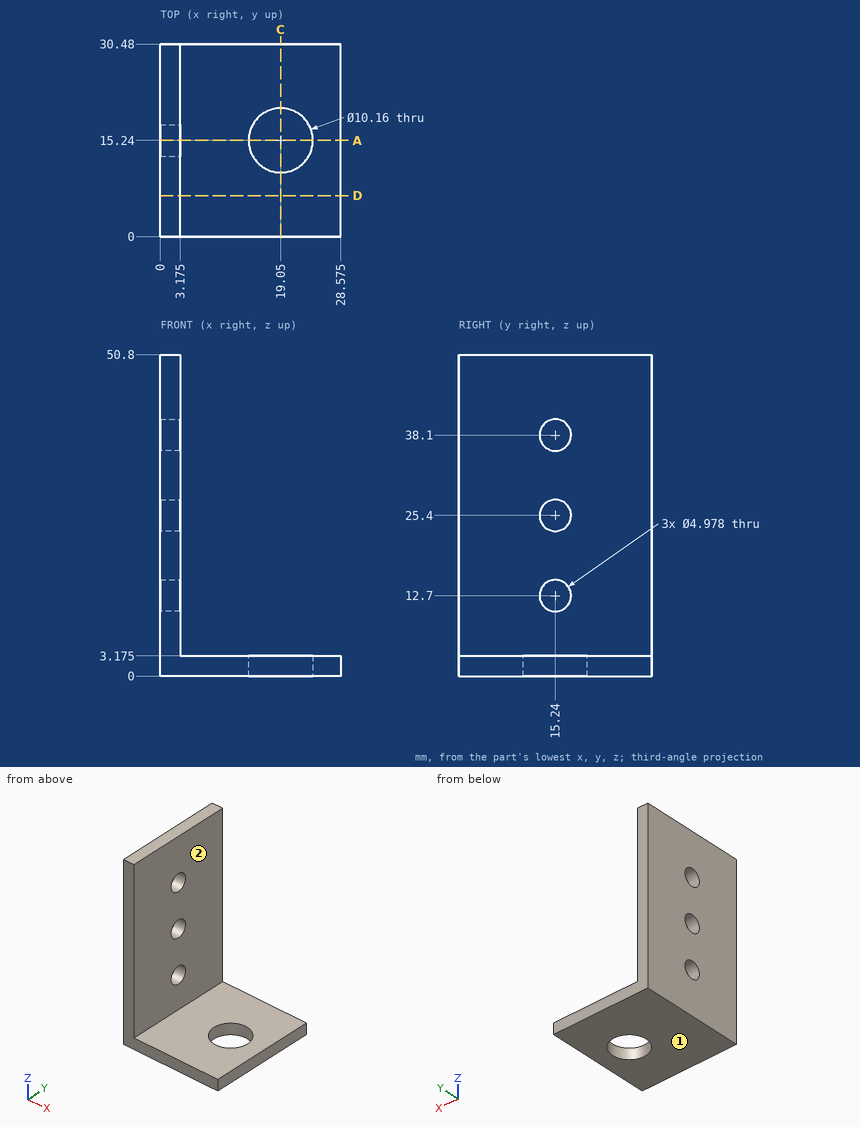
Job drawing, mm, ordinate dimensions from the low corner. One solid piece. A direction names the side the tool comes from. Round coordinates to 2 decimals unless told otherwise and drop trailing zeros. Loops run counter-clockwise (first coordinate to the right, second up) from the corner with the lowest first, then second, coordinate; pieces in that order, holes last. Notation, with made-up numbers: (-39.5, -14) -> (-19.5, -14) arc R16 cw to (-19.5, 13) -> close; hole circle Ø4 at (-36.5, 74.25). An arc over 180 degrees is marked (long way). One line per item, written item: value. Start each with the question number.
Q1. Drop flat-ended pins along their axis: pin 1 Ø4.5 at (y, z) = (15.24, 25.4) entering from -X; pin 2 Ø10 at (y, z) = (16, 34) entering from -X; pin 3 Ø7.5 at (x, y) = (20, 21) entering from +Z (3 decimals). Give the stop position or say it passes through.
Q2. Cut at D-D on y = 6.5. List the corners of the cut face in (x, z) (1 decimal), plus the area to 3 significant figures.
Q3. 3-axis set-ups, long thin cutter, end or side, ignore diameter. For the marked faces 1 and 2: which of +Z, -Z, +X, -X, +Y, -Y reach the whole face in a straight line?
Q4. Probe line 1 along Y through (x, z) = (0.8, 12.7); line 2 along X through (y, z) = (9, 46) (1 decimal); line 3 along Y through (x, z) = (19.05, 2.15). List the from-to ranges inside material, lowest first.
Q5. Cut at A-A on y = 15.24. List the corners of the cut face in (x, z) (1 decimal).
Q6. Cut at C-C on x = 19.05. List the corners of the cut face in (y, z) (1 decimal).
Computed:
1. pin 1: through
1. pin 2: x = 0
1. pin 3: z = 3.175
2. outline: (0, 0) -> (28.6, 0) -> (28.6, 3.2) -> (3.2, 3.2) -> (3.2, 50.8) -> (0, 50.8) -> close
2. area: 242 mm²
3. face 1: -Z, +X, -X, +Y, -Y
3. face 2: +Z, +X, +Y, -Y
4. line 1: 0 to 12.75, 17.73 to 30.48
4. line 2: 0 to 3.2
4. line 3: 0 to 10.16, 20.32 to 30.48
5. outline: (0, 0) -> (14, 0) -> (14, 3.2) -> (3.2, 3.2) -> (3.2, 10.2) -> (0, 10.2) -> close; (0, 15.2) -> (3.2, 15.2) -> (3.2, 22.9) -> (0, 22.9) -> close; (0, 27.9) -> (3.2, 27.9) -> (3.2, 35.6) -> (0, 35.6) -> close; (0, 40.6) -> (3.2, 40.6) -> (3.2, 50.8) -> (0, 50.8) -> close; (24.1, 0) -> (28.6, 0) -> (28.6, 3.2) -> (24.1, 3.2) -> close
6. outline: (0, 0) -> (10.2, 0) -> (10.2, 3.2) -> (0, 3.2) -> close; (20.3, 0) -> (30.5, 0) -> (30.5, 3.2) -> (20.3, 3.2) -> close
